Check sheet for the modelled part. Datum: model origin and axes. Units: mm. A direction names the side the tool comes from. Give positions to 0.01 mm unless a question says otherwise; leave off trailing zeros. Answer in a Markdown table with one row per item. Add a question column.
(1) Go/stop test with flat-tipped pins: pin 1 (1.5 mm diameter, centred on y = -27, z = -1.5, fed in from +X); pin 2 (1.5 mm diameter, centred on x = 28.5, z = -2, fed in from +Y); pin 3 (4 mm diameter, centred on y = -5, z = -3, fed in from -X). Record where each tip stops, or that it passes through.
(2) Thickness scan on L1, parallel to X at y = 35, z = 2. Record the ranges inside material, lowest first. Write a range as [from, to].
(3) Set-up check for faces 1 (the face through (-1, 59.69, -3)), 2 (the face through (-59.69, 1, -3)), 3 (the face through (-1, -59.69, -3)), 4 (the face through (59.69, 1, -3)): record each of +Z, -Z, +X, -X, +Y, -Y from which the full face is reachable in a straight line by a thin tool's end or side.
```python
from build123d import *

# Parameters (mm, degrees)
F0_W     = 127
F0_H     = 127
F1_DEPTH = 127
F2_W     = 119.38
F2_H     = 119.38
F3_DEPTH = 6.35
F4_R     = 2.54
F5_R     = 2.54
F6_R     = 1.27


with BuildPart() as f1:
    # F0 (on Top) → F1 (new body)
    with BuildSketch(Plane.XY):
        Rectangle(F0_W, F0_H)
    extrude(amount=F1_DEPTH)

    # F2 (on face) → F3 (join)
    with BuildSketch(Plane(origin=(0, 0, 0), x_dir=(1, 0, 0), z_dir=(0, 0, -1))):
        Rectangle(F2_W, F2_H)
    extrude(amount=F3_DEPTH)

    # F4
    f4_edges = [f1.edges().sort_by_distance(p)[0] for p in [
        (63.5, 63.5, 63.5),
        (-63.5, 63.5, 63.5),
        (0, 63.5, 0),
        (0, 63.5, 127),
        (-63.5, -63.5, 63.5),
        (-63.5, 0, 0),
        (-63.5, 0, 127),
        (63.5, -63.5, 63.5),
        (0, -63.5, 0),
        (0, -63.5, 127),
        (63.5, 0, 0),
        (63.5, 0, 127),
    ]]
    fillet(f4_edges, radius=F4_R)

    # F5
    f5_edges = [f1.edges().sort_by_distance(p)[0] for p in [
        (59.69, -59.69, -3.175),
        (-59.69, -59.69, -3.175),
        (59.69, 59.69, -3.175),
        (-59.69, 59.69, -3.175),
    ]]
    fillet(f5_edges, radius=F5_R)

    # F6
    f6_edges = [f1.edges().sort_by_distance(p)[0] for p in [
        (0, -59.69, -6.35),
        (58.946051, -58.946051, -6.35),
        (-58.946051, -58.946051, -6.35),
        (59.69, 0, -6.35),
        (-59.69, 0, -6.35),
        (58.946051, 58.946051, -6.35),
        (-58.946051, 58.946051, -6.35),
        (0, 59.69, -6.35),
    ]]
    fillet(f6_edges, radius=F6_R)


solid = f1.part
```
Answer below:
| question | item | result |
|---|---|---|
| 1 | pin 1 | stops at x = 59.69 |
| 1 | pin 2 | stops at y = 59.69 |
| 1 | pin 3 | stops at x = -59.69 |
| 2 | L1 | x = [-63.44, 63.44] |
| 3 | face 1 | -Z, +X, -X, +Y |
| 3 | face 2 | -Z, -X, +Y, -Y |
| 3 | face 3 | -Z, +X, -X, -Y |
| 3 | face 4 | -Z, +X, +Y, -Y |
